Source: CAD feature listing. Evaluate the final solid. Frame: model axes, mm. Face numbers are marked on the shaded views. A direction names the side the tool comes from. Give positions to 0.01 mm unless a question says otherwise; leave off trailing zeros. Write each loop counter-clockwise with the first axis right and the second up, starting at its lowest first coordinate (ties: lowest second). Pieces come first, ordered by that corner, then holes. Notation, with made-up numbers: M -28,-6.5 L 10,-6.5 A35 cw 10,27.5 Z; hole C 18,23.5 d1. An arc over 180 degrees is marked long. Return JSON: item names as keys, results as strings.
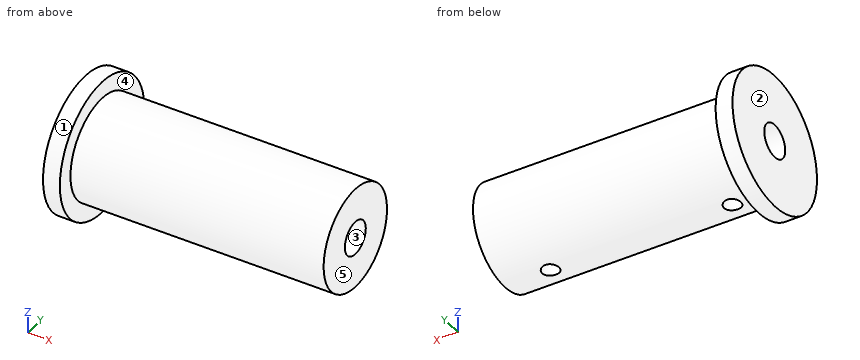
```python
from build123d import *

# Parameters (mm, degrees)
F2_R     = 0.5
F3_DEPTH = 4.001


# Not quite as in the source:
# - a feature names something its author has since deleted; it is built from what else it names


with BuildPart() as f1:
    # F0 (on Front) → F1 (revolve)
    with BuildSketch(Plane.XZ):
        Polygon((0, 4), (0, 0.99), (16, 0.99), (16, 3), (1, 3), (1, 4), align=None)
    revolve(axis=Axis((-1.1582460975, 0, 0), (1, 0, 0)))

    # F2 (on Top) → F3 (cut, through all)
    with BuildSketch(Plane.XY):
        with Locations((2.5, 0)):
            Circle(F2_R)
        with Locations((13.275148347, 0)):
            Circle(F2_R)
    extrude(amount=-F3_DEPTH, mode=Mode.SUBTRACT)


solid = f1.part
```
1) Line query: line 1 (X direction, y = 0, z = -1.5); line 2 (X direction, y = -3.5, z = -0.5); line 3 (Y direction, x = 11.5, z = -0.5). Output: solid intervals per line, ascending. Write a range as [from, to].
Numbers:
{"line 1": "x = [0, 2], [3, 12.78], [13.78, 16]", "line 2": "x = [0, 1]", "line 3": "y = [-2.96, -0.85], [0.85, 2.96]"}
2) Cut plane D-D, the plane y = -1.75. Return the cut outline in (x, z).
Numbers:
{"outline": "M 0,-3.6 L 1,-3.6 L 1,-2.44 L 16,-2.44 L 16,2.44 L 1,2.44 L 1,3.6 L 0,3.6 Z"}
3) Draft query along Z for the marked faces 1, 2 and 3. Return one class per face: released by +Z, released by -Z, zero draft, split by the parting line, or undercut.
Numbers:
{"face 1": "split by the parting line", "face 2": "zero draft", "face 3": "undercut"}
4) Cut plane A-A, the plane y = 0. Return the cut outline in (x, z).
Numbers:
{"outline": "M 0,-4 L 1,-4 L 1,-3 L 2,-3 L 2,-0.99 L 0,-0.99 Z; M 0,0.99 L 16,0.99 L 16,3 L 1,3 L 1,4 L 0,4 Z; M 3,-3 L 12.78,-3 L 12.78,-0.99 L 3,-0.99 Z; M 13.78,-3 L 16,-3 L 16,-0.99 L 13.78,-0.99 Z"}
5) Contact query for flat-ended pins moving along their axis: pin 1 Ø2 at (x, y) = (10, 2.5) entering from -Z; pin 2 Ø1.5 at (x, y) = (9, -3) entering from -Z. Output: stop coordinate, or through.
Numbers:
{"pin 1": "stops at z = -2.6", "pin 2": "stops at z = -1.98"}
6) Cut plane C-C, the plane z = -2.5. Return the cut outline in (x, y).
Numbers:
{"outline": "M 0,-3.12 L 1,-3.12 L 1,-1.66 L 16,-1.66 L 16,1.66 L 1,1.66 L 1,3.12 L 0,3.12 Z; hole C 2.5,0 d1; hole C 13.28,0 d1"}
7) Set-up query: the marked faces 4 and 5. Return all of +Z, -Z, +X, -X, +Y, -Y with unobstructed straight access to the full face (end or side cutting, diameter ignored); none if empty.
Numbers:
{"face 4": "+X", "face 5": "+Z, -Z, +X, +Y, -Y"}
8) Cut plane B-B, the plane z = 0.75. Return the cut outline in (x, y), then the cut area to 3 significant figures.
Numbers:
{"outline": "M 0,-3.93 L 1,-3.93 L 1,-2.9 L 16,-2.9 L 16,-0.65 L 0,-0.65 Z; M 0,0.65 L 16,0.65 L 16,2.9 L 1,2.9 L 1,3.93 L 0,3.93 Z", "area": "74.3 mm²"}
